from build123d import *

# Parameters (mm, degrees)
F1_DEPTH      = 10
F3_W          = 4.8
F3_H          = 5
F4_DEPTH      = 5
F5_W          = 3
F5_H          = 3
F6_DEPTH      = 2.5
F7_R          = 1
F8_R          = 1
F9_R          = 1
F10_R         = 1
F11_R         = 1
F12_T1_DEPTH  = 33.1967746272
F12_T3_DEPTH  = 8
F12_T8_DEPTH  = 1
F12_T14_DEPTH = 1
F13_T1_DEPTH  = 26.4086914989
F13_T3_DEPTH  = 8
F13_T8_DEPTH  = 1
F13_T14_DEPTH = 1


# Not quite as in the source:
# - a fillet or chamfer that OpenCascade refuses, or shapes differently, is made with other operations: its cross-section is extruded or revolved along the edge and cut away or added


with BuildPart() as f1:
    # F0 (on Front) → F1 (new body)
    with BuildSketch(Plane.XZ):
        Polygon((25, 0), (0, 0), (0, -7), (31.589826983, -68.1461583276), (42.589826983, -68.1461583276), (42.589826983, -36.1461583276), (21.3394588046, -41.8401773199), align=None)
    extrude(amount=F1_DEPTH)

    # F3 (on face) → F4 (join)
    with BuildSketch(Plane(origin=(0, 0, -68.1461583276), x_dir=(1, 0, 0), z_dir=(0, 0, -1))):
        with Locations((37.089826983, 5)):
            Rectangle(F3_W, F3_H)
    extrude(amount=F4_DEPTH)

    # F5 (on face) → F6 (cut)
    with BuildSketch(Plane(origin=(0, 0, 0), x_dir=(0, -1, 0), z_dir=(-1, 0, 0))):
        with Locations((5, -3.5)):
            Rectangle(F5_W, F5_H)
    extrude(amount=-F6_DEPTH, mode=Mode.SUBTRACT)

    # F7
    f7_edges = [f1.edges().sort_by_distance(p)[0] for p in [
        (23.169729, -10, -20.920089),
    ]]
    fillet(f7_edges, radius=F7_R)

    # F8
    f8_edges = [f1.edges().sort_by_distance(p)[0] for p in [
        (23.169729, 0, -20.920089),
    ]]
    fillet(f8_edges, radius=F8_R)

    # F9
    f9_edges = [f1.edges().sort_by_distance(p)[0] for p in [
        (15.794913, 0, -37.573079),
        (15.794913, -10, -37.573079),
    ]]
    fillet(f9_edges, radius=F9_R)

    # F10
    f10_edges = [f1.edges().sort_by_distance(p)[0] for p in [
        (31.964643, 0, -38.993168),
    ]]
    fillet(f10_edges, radius=F10_R)

    # F11
    f11_edges = [f1.edges().sort_by_distance(p)[0] for p in [
        (31.964643, -10, -38.993168),
    ]]
    fillet(f11_edges, radius=F11_R)

    # F12: fillet of radius 1 on 1 edges, made by hand

    # F12_s2 → F12_t1 (cut)
    with BuildSketch(Plane.XY.offset(-70.6461583276)):
        with BuildLine():
            ThreePointArc((42.589826983, -1), (42.2969337641, -0.2928932188), (41.589826983, 0))
            Line((41.589826983, 0), (42.589826983, 0))
            Line((42.589826983, 0), (42.589826983, -1))
        make_face()
        with BuildLine():
            ThreePointArc((42.589826983, -9), (42.2969337641, -9.7071067812), (41.589826983, -10))
            Line((41.589826983, -10), (42.589826983, -10))
            Line((42.589826983, -10), (42.589826983, -9))
        make_face()
    extrude(amount=F12_T1_DEPTH, mode=Mode.SUBTRACT)

    # F12_s4 → F12_t3 (cut)
    with BuildSketch(Plane.XZ.offset(1)):
        with BuildLine():
            ThreePointArc((42.589826983, -37.4493837004), (42.198588412, -36.6560303601), (41.3310079379, -36.4834578742))
            Line((41.3310079379, -36.4834578742), (42.589826983, -36.1461583276))
            Line((42.589826983, -36.1461583276), (42.589826983, -37.4493837004))
        make_face()
    extrude(amount=F12_T3_DEPTH, mode=Mode.SUBTRACT)


with BuildPart() as f12_tool6:
    # F12_s7 → F12_t8 (new body)
    with BuildSketch(Plane.XZ.offset(1)):
        Polygon((41.589826983, -37.4493837004), (42.589826983, -37.4493837004), (42.589826983, -36.1461583276), (41.3310079379, -36.4834578742), align=None)
    extrude(amount=-F12_T8_DEPTH)

    # F12_s9 → F12_t10 (revolve, cut)
    with BuildSketch(Plane(origin=(41.589826983, -1, -37.4493837004), x_dir=(-0.608761429, 0, -0.7933533403), z_dir=(0.7933533403, 0, -0.608761429))):
        with BuildLine():
            ThreePointArc((0, -1), (1, 0), (0, 1))
            Line((0, 1), (0, -1))
        make_face()
    revolve(axis=Axis((41.589826983, -1, -37.4493837004), (0, 1, 0)), mode=Mode.SUBTRACT)


with BuildPart() as f1_1:
    add(f1.part)

    # F12_t5: cut F12_tool6
    add(f12_tool6.part, mode=Mode.SUBTRACT)


with BuildPart() as f12_tool12:
    # F12_s13 → F12_t14 (new body)
    with BuildSketch(Plane.XZ.offset(9)):
        Polygon((41.589826983, -37.4493837004), (42.589826983, -37.4493837004), (42.589826983, -36.1461583276), (41.3310079379, -36.4834578742), align=None)
    extrude(amount=F12_T14_DEPTH)

    # F12_s15 → F12_t16 (revolve, cut)
    with BuildSketch(Plane(origin=(41.589826983, -9, -37.4493837004), x_dir=(-0.608761429, 0, -0.7933533403), z_dir=(-0.7933533403, 0, 0.608761429))):
        with BuildLine():
            ThreePointArc((0, -1), (1, 0), (0, 1))
            Line((0, 1), (0, -1))
        make_face()
    revolve(axis=Axis((41.589826983, -9, -37.4493837004), (0, -1, 0)), mode=Mode.SUBTRACT)


with BuildPart() as f1_2:
    add(f1_1.part)

    # F12_t11: cut F12_tool12
    add(f12_tool12.part, mode=Mode.SUBTRACT)

    # F13: fillet of radius 1 on 3 edges, made by hand

    # F13_s2 → F13_t1 (cut)
    with BuildSketch(Plane.YZ.offset(-2.5)):
        with BuildLine():
            ThreePointArc((-10, -1), (-9.7071067812, -0.2928932188), (-9, 0))
            Line((-9, 0), (-10, 0))
            Line((-10, 0), (-10, -1))
        make_face()
        with BuildLine():
            ThreePointArc((-1, 0), (-0.2928932188, -0.2928932188), (0, -1))
            Line((0, -1), (0, 0))
            Line((0, 0), (-1, 0))
        make_face()
    extrude(amount=F13_T1_DEPTH, mode=Mode.SUBTRACT)

    # F13_s4 → F13_t3 (cut)
    with BuildSketch(Plane.XZ.offset(1)):
        with BuildLine():
            ThreePointArc((24.904886197, -1.0871557427), (24.6459688357, -0.3244097924), (23.9086914989, 0))
            Line((23.9086914989, 0), (25, 0))
            Line((25, 0), (24.904886197, -1.0871557427))
        make_face()
    extrude(amount=F13_T3_DEPTH, mode=Mode.SUBTRACT)


with BuildPart() as f13_tool6:
    # F13_s7 → F13_t8 (new body)
    with BuildSketch(Plane.XZ.offset(1)):
        Polygon((23.9086914989, -1), (24.904886197, -1.0871557427), (25, 0), (23.9086914989, 0), align=None)
    extrude(amount=-F13_T8_DEPTH)

    # F13_s9 → F13_t10 (revolve, cut)
    with BuildSketch(Plane(origin=(23.9086914989, -1, -1), x_dir=(-0.7372773368, 0, -0.6755902076), z_dir=(0.6755902076, 0, -0.7372773368))):
        with BuildLine():
            ThreePointArc((0, -1), (1, 0), (0, 1))
            Line((0, 1), (0, -1))
        make_face()
    revolve(axis=Axis((23.9086914989, -1, -1), (0, 1, 0)), mode=Mode.SUBTRACT)


with BuildPart() as f1_3:
    add(f1_2.part)

    # F13_t5: cut F13_tool6
    add(f13_tool6.part, mode=Mode.SUBTRACT)


with BuildPart() as f13_tool12:
    # F13_s13 → F13_t14 (new body)
    with BuildSketch(Plane.XZ.offset(9)):
        Polygon((23.9086914989, -1), (24.904886197, -1.0871557427), (25, 0), (23.9086914989, 0), align=None)
    extrude(amount=F13_T14_DEPTH)

    # F13_s15 → F13_t16 (revolve, cut)
    with BuildSketch(Plane(origin=(23.9086914989, -9, -1), x_dir=(-0.7372773368, 0, -0.6755902076), z_dir=(-0.6755902076, 0, 0.7372773368))):
        with BuildLine():
            ThreePointArc((0, -1), (1, 0), (0, 1))
            Line((0, 1), (0, -1))
        make_face()
    revolve(axis=Axis((23.9086914989, -9, -1), (0, -1, 0)), mode=Mode.SUBTRACT)


with BuildPart() as f1_4:
    add(f1_3.part)

    # F13_t11: cut F13_tool12
    add(f13_tool12.part, mode=Mode.SUBTRACT)


solid = f1_4.part
Here's how the part is built. I have some questions about the finished solid (model axes, mm). A direction names the side the tool comes from. Give positions to 0.01 mm unless a question says otherwise; leave off trailing zeros. Loops run counter-clockwise (first coordinate to the right, second up) from the corner with the lowest first, then second, coordinate; pieces in that order, holes last. Notation, with made-up numbers: (82.5, 20) -> (96.5, 20) arc R11 cw to (96.5, 26) -> close; hole circle Ø10 at (30, -32). An arc over 180 degrees is marked (long way). One line per item, written item: value.
Q1. I'm going to push flat-ended pins straight in: pin 1 Ø2 at (x, y) = (1, -4.5) entering from -Z; pin 2 Ø4 at (x, z) = (37.5, -71.5) entering from -Y; pin 3 Ø6 at (x, y) = (25.5, -9) entering from +Z; pin 4 Ø0.9 at (y, z) = (-4.5, -3) entering from -X. Where does each tip first touch, or does it pass through?
Answers follow:
pin 1: z = -10.87
pin 2: y = -7.5
pin 3: z = 0
pin 4: x = 2.5
Q2. Suppose I cut it at A-A on y = -4.75. Please give me the cut outline in (x, z), then the cut area to 3 significant figures.
Answers follow:
outline: (0, -7) -> (31.59, -68.15) -> (34.69, -68.15) -> (34.69, -73.15) -> (39.49, -73.15) -> (39.49, -68.15) -> (42.59, -68.15) -> (42.59, -37.45) arc R1 ccw to (41.33, -36.48) -> (21.34, -41.84) -> (24.9, -1.09) arc R1 ccw to (23.91, 0) -> (0, 0) -> (0, -2) -> (2.5, -2) -> (2.5, -5) -> (0, -5) -> close
area: 1,200 mm^2
Q3. If I drill on line 1 along X through (y, z) = (-3.75, -49.5); line 2 along Z through (x, y) = (17.5, -5.75); line 3 along Z through (x, y) = (20, -0.75), over which ranges is the centre line in solid material (lowest first)?
Answers follow:
line 1: 21.96 to 42.59
line 2: -40.87 to 0
line 3: -45.64 to -0.03
Q4. On a 3-axis mill with a long thin cutter (end or side, diameter ignored), from which of +Z, -Z, +X, -X, +Y, -Y can I reach the whole of each face in a straight line? I mean faces 1 (the face through (37, -7.5, -71)), 2 (the face through (39.49, -5, -71)), 3 (the face through (30.574, -9.715, -39.677)). Say none if no direction works.
Answers follow:
face 1: -Z, +X, -X, -Y
face 2: -Z, +X, +Y, -Y
face 3: -Y
Q5. We'd pull the mould along Y, two halves only. Please class faces 4 (the face through (34.69, -5, -71)), 5 (the face through (37, -2.5, -71)), 6 (the face through (1, -5, -2)), 7 (the face through (1, -3.5, -4)): pulls with the +Y half, pulls with the -Y half, needs draft (parallel to the pull), parting line crosses it, or undercut.
Answers follow:
face 4: needs draft
face 5: pulls with the +Y half
face 6: undercut
face 7: undercut
